from build123d import *

# Parameters (mm, degrees)
F2_R            = 7.5
F3_DEPTH        = 12.701
F3_COPIES_COUNT = 6
F4_W            = 14.403924346
F4_H            = 14.403924346
F5_DEPTH        = 12.701


# Not quite as in the source:
# - a pattern or mirror of a feature is missing from the dataset's text; its kind, count and spacing are read off the source's solid


with BuildPart() as f1:
    # F0 (on Front) → F1 (revolve)
    with BuildSketch(Plane.XZ):
        Polygon((25.4, 60.325), (12.7, 60.325), (12.7, 34.6970452561), (32.7323484187, 0), (63.5, 0), (63.5, 12.7), (40.0646968374, 12.7), (25.4, 38.1), align=None)
    revolve(axis=Axis((0, 0, 18.9653343184), (0, 0, 1)))

    # F2 (on face) → F3 (cut, through all)
    with BuildSketch(Plane.XY.offset(12.7)):
        with Locations((-50.8, 0)):
            Circle(F2_R)
    f3 = extrude(amount=-F3_DEPTH, mode=Mode.SUBTRACT)

    # F3_copies: F3 ×6 about axis
    f3_copies_axis = Axis((0, 0, 0), (0, 0, 1))
    for i in range(1, F3_COPIES_COUNT):
        add(f3.rotate(f3_copies_axis, i * 360 / F3_COPIES_COUNT), mode=Mode.SUBTRACT)

    # F4 (on face) → F5 (cut, through all)
    with BuildSketch(Plane.XY.offset(12.7)):
        with Locations((0, -51.4825247228)):
            Rectangle(F4_W, F4_H)
    extrude(amount=-F5_DEPTH, mode=Mode.SUBTRACT)


solid = f1.part
Geometry check sheet. Reference: the model listing, model coordinates, mm. A direction names the side the tool comes from. Give positions to 0.01 mm unless a question says otherwise; leave off trailing zeros. Write each loop counter-clockwise with the first axis right and the second up, starting at its lowest first coordinate (ties: lowest second). Pieces come first, ordered by that corner, then holes. Notation, with made-up numbers: M 4.25,-21.75 L 37.25,-21.75 A24 ccw 37.25,10.25 Z; hole C 29,26.25 d4. An arc over 180 degrees is marked long. Answer as CSV lines item,"result". Start each with the question number.
Q1. Section check A-A, the plane x = 50.8. Record the cut outline in (y, z).
Q2. Section check D-D, the plane z = 29.5. Record the cut outline in (x, y).
Q3. Material ranges on L1, parallel to Y at x = 25.4, z = 9.25; L2, parallel to Y at x = 25.4, z = 5.5; L3, parallel to Z at x = 56.5, y = 24.5, recorded low to high.
Q4. Release check for a two-part mould opening along X. For faces 1 (the face through (-13.77, -61.99, 6.44)), 2 (the face through (17.907, -43.664, 6.439)), 3 (the face through (-27, -27, 0)) record: pulls with the +X half, pulls with the -X half, needs draft (parallel to the pull), parting line crosses it, or undercut.
Q5. Section check B-B, the plane y = 0. Record the cut outline in (x, z) (3 decimals).
Q6. Tool access check on faces 4 (the face through (-5.506, -24.796, 49.368)), 5 (the face through (5, 12, 60.325)), 6 (the face through (0, -58.684, 6)). Record the directions out of +Z, -Z, +X, -X, +Y, -Y that give a thin tool (end or side, any length) a straight path to the whole face; none if there is none.
Q7. Section check C-C, the plane x = -54. Record the cut outline in (y, z).
Q8. Go/stop test with flat-tipped pins: pin 1 (10 mm diameter, centred on y = 14.5, z = 43, fed in from -X); pin 2 (6.5 mm diameter, centred on x = -2.5, z = 8.5, fed in from -Y); pin 3 (4 mm diameter, centred on y = -48, z = 3.5, fed in from +X) (3 decimals); pin 4 (15 mm diameter, centred on x = 0, y = 0, fed in from +Z). Record where each tip stops, or that it passes through.
Geometry says:
1,outline,"M -38.1,0 L -7.5,0 L -7.5,12.7 L -38.1,12.7 Z; M 7.5,0 L 38.1,0 L 38.1,12.7 L 7.5,12.7 Z"
2,outline,"C 0,0 d60.73; hole C 0,0 d31.4"
3,L1,"-58.2 to -51.49, -36.49 to -10.25, 10.25 to 36.49, 51.49 to 58.2"
3,L2,"-58.2 to -51.49, -36.49 to -15.11, 15.11 to 36.49, 51.49 to 58.2"
3,L3,"0 to 12.7"
4,face 1,"parting line crosses it"
4,face 2,"undercut"
4,face 3,"needs draft"
5,outline,"M -63.5,0 L -58.3,0 L -58.3,12.7 L -63.5,12.7 Z; M -43.3,0 L -32.732,0 L -12.7,34.697 L -12.7,60.325 L -25.4,60.325 L -25.4,38.1 L -40.065,12.7 L -43.3,12.7 Z; M 12.7,34.697 L 32.732,0 L 43.3,0 L 43.3,12.7 L 40.065,12.7 L 25.4,38.1 L 25.4,60.325 L 12.7,60.325 Z; M 58.3,0 L 63.5,0 L 63.5,12.7 L 58.3,12.7 Z"
6,face 4,"+Z"
6,face 5,"+Z, +X, -X, +Y, -Y"
6,face 6,"+Z, -Z"
7,outline,"M -33.41,0 L -6.78,0 L -6.78,12.7 L -33.41,12.7 Z; M 6.78,0 L 33.41,0 L 33.41,12.7 L 6.78,12.7 Z"
8,pin 1,"x = -23.56"
8,pin 2,"y = -63.5"
8,pin 3,"x = 43.775"
8,pin 4,"through"
